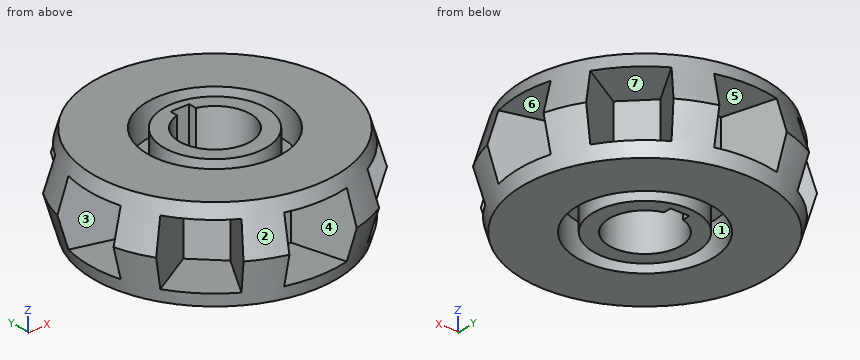
Autodesk Inventor part; units mm, degrees
ref_plane "YZ Plane" through (0, 0, 0) normal (1, 0, 0) x (0, 1, 0)
ref_plane "XZ Plane" through (0, 0, 0) normal (0, 1, 0) x (-1, 0, 0)
ref_plane "XY Plane" through (0, 0, 0) normal (0, 0, 1) x (1, 0, 0)
sketch "Sketch1" plane through (0, 0, 0) normal (0, 0, 1) x (1, 0, 0)
  circle A0 centre (0, 0) radius 22.5
  dimension "d0" = 45
extrude "Extrusion1" add sketch "Sketch1" along normal mid plane 17
sketch "Sketch2" plane through (0, 0, 8.5) normal (0, 0, 1) x (1, 0, 0)
  circle A0 centre (0, 0) radius 6.6
  line L0 (-1.75, 7.8638) -> (1.75, 7.8638)
  line L1 (1.75, 7.8638) -> (1.75, 6.3638)
  line L2 (1.75, 6.3638) -> (-1.75, 6.3638)
  line L3 (-1.75, 6.3638) -> (-1.75, 7.8638)
  dimension "d3" = 13.2
  dimension "d4" = 3.5
  dimension "d5" = 1.5
extrude "Extrusion2" cut sketch "Sketch2" against normal through all
sketch "Sketch3" plane through (0, 0, 8.5) normal (0, 0, 1) x (1, 0, 0)
  circle A0 centre (0, 0) radius 9.5
  circle A1 centre (0, 0) radius 12.5
  dimension "d8" = 19
  dimension "d9" = 3
extrude "Extrusion3" cut sketch "Sketch3" against normal blind 6
mirror "Mirror1" about plane through (0, 0, 0) normal (0, 0, 1) of "Extrusion3"
sketch "Sketch4" plane through (0, 0, 0) normal (0, 1, 0) x (-1, 0, 0)
  line L0 (22.5, -8.5) -> (22.5, 8.5)
  line L1 (22.5, -8.5) -> (25, 0)
  line L2 (25, 0) -> (22.5, 8.5)
  line L3 (-22.5, -8.5) -> (22.5, -8.5)
  line L4 (34.5, 0) -> (-32, 0)
  line L5 (0, -11.9) -> (0, 11.9)
  point P0 (0, 0)
  dimension "d12" = 2.5
revolve "Revolution1" add sketch "Sketch4" angle 360 about axis through (0, 0, -10) along (0, 0, 1) contours L0 L4 L1 | L0 L2 L4
sketch "Sketch5" plane through (0, 0, 0) normal (0, 0, 1) x (1, 0, 0)
  line L0 (-6.5, 25) -> (-3.38, 13)
  line L1 (-3.38, 13) -> (3.38, 13)
  line L2 (3.38, 13) -> (6.5, 25)
  line L3 (6.5, 25) -> (-6.5, 25)
  circle A0 centre (0, 0) radius 25 construction
  line L4 (0, -35) -> (0, 35) construction
  point P0 (0, 13)
  point P1 (0, 25)
  dimension "d14" = 13
  dimension "d15" = 12
extrude "Extrusion4" cut sketch "Sketch5" along normal mid plane 12
pattern_circular "Circular Pattern1" count 8 over 360 about axis through (0, 0, -10) along (0, 0, 1) of "Extrusion4"
sketch "Sketch6" plane through (0, 0, 0) normal (0, 0, 1) x (1, 0, 0)
  circle A0 centre (0, 0) radius 20.5
  dimension "d21" = 41
properties part number "omniwheel"
Build history of the part. All positions in model axes, mm. Face numbers are marked on the shaded views. A direction names the side the tool comes from. Give positions to 0.01 mm unless a question says otherwise; leave off trailing zeros. One line per question, with ' | ' between items. Start each with the question number.
1) Cut at C-C (z = -3.5). Count the separate pieces of the cut face and the enclosed holes in it, plus the area to 4 significant figures.
2) Two-plate mould, pull along Z, no slides. Class the marked faces 1, 2 and 3: released by +Z, released by -Z, zero draft, split by the parting line, or undercut.
3) 3-axis set-ups, long thin cutter, end or side, ignore diameter. For the marked faces 4, 5, 6 and 7: which of +Z, -Z, +X, -X, +Y, -Y reach the whole face in a straight line?
4) Probe L1, parallel to Y at x = 0, z = -4.25; L2, parallel to Y at x = 11.5, z = -1; L3, parallel to X at y = 8.5, z = -5.75. List the from-to ranges inside material, lowest first.
5) Pin check, flat tips, straight feed: pin 1 (4 mm diameter, centred on x = -12, z = -1, fed in from +Y); pin 2 (1.2 mm diameter, centred on y = 7, z = 0, fed in from +X); pin 3 (5 mm diameter, centred on x = -9.5, z = 6.5, fed in from -Y). Stop position of each tip, or through.
Return value:
1) separate pieces: 2 | enclosed holes: 2 | area: 638.5 mm^2
2) face 1: zero draft | face 2: released by +Z | face 3: undercut
3) face 4: -Y | face 5: +Y | face 6: +X | face 7: none
4) L1: -13 to -12.5, -9.5 to -6.6, 7.86 to 9.5, 12.5 to 13 | L2: -21.87 to -19.58, -6.88 to 6.88, 19.58 to 21.87 | L3: -21.7 to -14.47, -9.88 to -9.17, -4.24 to 4.24, 9.17 to 9.88, 14.47 to 21.7
5) pin 1: y = 22.79 | pin 2: x = 24.17 | pin 3: y = -22.31
